Could you check a few things on this model? Use its own coordinates, in mm. A direction names the side the tool comes from. Give positions to 0.01 mm unless a question says otherwise; leave off trailing zeros. Loops run counter-clockwise (first coordinate to the right, second up) from the corner with the lowest first, then second, coordinate; pieces in that order, holes last. Notation, with made-up numbers: (-34.5, 64) - (-8.5, 64) arc R15 ccw to (-8.5, 77) - close; hole circle Ø2 at (79, 30). An arc over 180 degrees is marked (long way). One line per item, written item: value. Start each with the question number.
Q1. If I drill on line 1 (Y direction, x = -8, z = 16.75); line 2 (Y direction, x = 67, z = 16.25) (3 decimals); line 3 (Z direction, x = 69.5, y = 14) (3 decimals), over which ranges is the centre line in solid material (lowest first)? Write a range as from..to.
Q2. I want a section at A-A (x = -33). Please give me the cut outline in (y, z), then the cut area to 3 significant figures.
Q3. I'm going to push flat-ended pins straight in: P1, Ø9, axis at x = -65.88, y = -2.54, coming from the -Z side; P2, Ø11.5, axis at x = -3, y = 2, coming from the +Z side; P3, Ø3, axis at y = 7.5, z = 10, coming from the -X side. Where does each tip first touch, or does it pass through?
Q4. For faces 4 (the face through (-60.74, -20.54, 10.32)), 5 (the face through (63.182, -11, 10)), 6 (the face through (0, 0, 3.429)), 7 (the face through (-72, 16, 3.175)), 8 (the face through (70, 10.033, 10)), which set-ups out of +Z, -Z, +X, -X, +Y, -Y let a thin tool reach every point of the face, with its end or its side?
Q5. I want a section at B-B (y = -18). Please give me the cut outline in (x, z) (3 decimals), then the cut area to 3 significant figures.
Q6. If we mould it in two halves opening along X, with no side actions, what happens to faces 1 (the face through (-63.182, -12, 10)), 2 (the face through (-70, 10.033, 10)), 3 (the face through (2, 19.494, 10))? For each: released by +X, released by -X, zero draft, split by the parting line, or undercut.
Q7. I want a section at D-D (y = 17). Please give me the cut outline in (x, z) (3 decimals), then the cut area to 3 significant figures.
Q8. I want a section at C-C (z = 9.5). Count the separate pieces of the cut face and the enclosed holes in it, then the cut area to 3 significant figures.
```python
from build123d import *

# Parameters (mm, degrees)
F1_DEPTH       = 17.272
F3_DEPTH       = 13.843
F5_DEPTH       = 14.097
F7_D           = 6.858
F7_CBORE_D     = 10.033
F7_CBORE_DEPTH = 3.048


# Not quite as in the source:
# - a feature names something its author has since deleted; it is built from what else it names


with BuildPart() as f1:
    # F0 (on Top) → F1 (new body)
    with BuildSketch(Plane.XY):
        with BuildLine():
            Line((68.0447455007, 22.86), (-68.0447455007, 22.86))
            ThreePointArc((-68.0447455007, 22.86), (-75.0673121338, 19.7699967275), (-77.5335, 12.5048415503))
            Line((-77.5335, 12.5048415503), (-75.2001773438, -14.1651584497))
            ThreePointArc((-75.2001773438, -14.1651584497), (-72.146419572, -20.3575666331), (-65.7114228444, -22.86))
            Line((-65.7114228444, -22.86), (70.3780681569, -22.86))
            ThreePointArc((70.3780681569, -22.86), (77.40063479, -19.7699967275), (79.8668226562, -12.5048415503))
            Line((79.8668226562, -12.5048415503), (77.5335, 14.1651584497))
            ThreePointArc((77.5335, 14.1651584497), (74.4797422282, 20.3575666331), (68.0447455007, 22.86))
        make_face()
    extrude(amount=F1_DEPTH)

    # F2 (on face) → F3 (cut)
    with BuildSketch(Plane.XY.offset(17.272)):
        with BuildLine():
            Line((56.1975, 19.4945), (-54.61, 19.4945))
            ThreePointArc((-54.61, 19.4945), (-57.9775960454, 18.0995960454), (-59.3725, 14.732))
            Line((-59.3725, 14.732), (-59.3725, -14.732))
            ThreePointArc((-59.3725, -14.732), (-57.9775960454, -18.0995960454), (-54.61, -19.4945))
            Line((-54.61, -19.4945), (56.1975, -19.4945))
            ThreePointArc((56.1975, -19.4945), (59.5650960454, -18.0995960454), (60.96, -14.732))
            Line((60.96, -14.732), (60.96, 14.732))
            ThreePointArc((60.96, 14.732), (59.5650960454, 18.0995960454), (56.1975, 19.4945))
        make_face()
    extrude(amount=-F3_DEPTH, mode=Mode.SUBTRACT)

    # F4 (on face) → F5 (cut)
    with BuildSketch(Plane.XY.offset(17.272)):
        with BuildLine():
            Line((-76.239581844, -2.2847106486), (-77.4044675129, 11.0299934736))
            ThreePointArc((-77.4044675129, 11.0299934736), (-77.4182058621, 11.1343465964), (-77.4227969589, 11.2395))
            Line((-77.4227969589, 11.2395), (-77.5335, 12.5048415503))
            ThreePointArc((-77.5335, 12.5048415503), (-77.0333154818, 16.4863861544), (-74.9377505887, 19.9085915493))
            ThreePointArc((-74.9377505887, 19.9085915493), (-71.7938897692, 22.0911145638), (-68.0447455007, 22.86))
            Line((-68.0447455007, 22.86), (-80.5285722017, 22.86))
            Line((-80.5285722017, 22.86), (-80.5285722017, -22.86))
            Line((-80.5285722017, -22.86), (-65.7114228444, -22.86))
            ThreePointArc((-65.7114228444, -22.86), (-72.146419572, -20.3575666331), (-75.2001773438, -14.1651584497))
            Line((-75.2001773438, -14.1651584497), (-76.1550120261, -3.2513480896))
            ThreePointArc((-76.1550120261, -3.2513480896), (-76.2140031856, -2.7694909766), (-76.239581844, -2.2847106486))
        make_face()
        with BuildLine():
            Line((-77.5335, 12.5048415503), (-77.4227969589, 11.2395))
            ThreePointArc((-77.4227969589, 11.2395), (-77.0694212904, 12.0926243315), (-76.2162969589, 12.446))
            Line((-76.2162969589, 12.446), (-70.4215, 12.446))
            ThreePointArc((-70.4215, 12.446), (-67.1195, 15.748), (-70.4215, 19.05))
            Line((-70.4215, 19.05), (-74.5701236506, 19.05))
            ThreePointArc((-74.5701236506, 19.05), (-75.0371164274, 19.358045639), (-74.9377505887, 19.9085915493))
            ThreePointArc((-74.9377505887, 19.9085915493), (-77.0333154818, 16.4863861544), (-77.5335, 12.5048415503))
        make_face()
        with BuildLine():
            Line((-63.1825, 3.81), (-63.1825, 10.033))
            Line((-63.1825, 10.033), (-76.2162969589, 10.033))
            ThreePointArc((-76.2162969589, 10.033), (-76.9918202099, 10.3152673794), (-77.4044675129, 11.0299934736))
            Line((-77.4044675129, 11.0299934736), (-76.239581844, -2.2847106486))
            ThreePointArc((-76.239581844, -2.2847106486), (-75.3866698867, 1.2003753653), (-72.9243249481, 3.81))
            Line((-72.9243249481, 3.81), (-63.1825, 3.81))
        make_face()
        with BuildLine():
            ThreePointArc((-72.7051694123, -8.255), (-74.9990780637, -6.1454708758), (-76.1550120261, -3.2513480896))
            Line((-76.1550120261, -3.2513480896), (-75.2001773438, -14.1651584497))
            ThreePointArc((-75.2001773438, -14.1651584497), (-72.146419572, -20.3575666331), (-65.7114228444, -22.86))
            Line((-65.7114228444, -22.86), (-55.0545, -22.86))
            ThreePointArc((-55.0545, -22.86), (-60.8018639175, -20.4793639175), (-63.1825, -14.732))
            Line((-63.1825, -14.732), (-63.1825, -8.255))
            Line((-63.1825, -8.255), (-72.7051694123, -8.255))
        make_face()
        with BuildLine():
            ThreePointArc((63.1825, -14.732), (60.8018639175, -20.4793639175), (55.0545, -22.86))
            Line((55.0545, -22.86), (70.3780681569, -22.86))
            ThreePointArc((70.3780681569, -22.86), (77.40063479, -19.7699967275), (79.8668226562, -12.5048415503))
            Line((79.8668226562, -12.5048415503), (78.9578200825, -2.114894589))
            ThreePointArc((78.9578200825, -2.114894589), (77.1524285249, -6.5300931701), (72.7051694123, -8.255))
            Line((72.7051694123, -8.255), (63.1825, -8.255))
            Line((63.1825, -8.255), (63.1825, -14.732))
        make_face()
        with BuildLine():
            ThreePointArc((77.5335, 14.1651584497), (76.7244498583, 17.2577996716), (74.9377505887, 19.9085915493))
            ThreePointArc((74.9377505887, 19.9085915493), (75.0371164274, 19.358045639), (74.5701236506, 19.05))
            Line((74.5701236506, 19.05), (70.4215, 19.05))
            ThreePointArc((70.4215, 19.05), (67.1195, 15.748), (70.4215, 12.446))
            Line((70.4215, 12.446), (76.2162969589, 12.446))
            ThreePointArc((76.2162969589, 12.446), (77.4227969589, 11.2395), (76.2162969589, 10.033))
            Line((76.2162969589, 10.033), (63.1825, 10.033))
            Line((63.1825, 10.033), (63.1825, 3.81))
            Line((63.1825, 3.81), (72.9243249481, 3.81))
            ThreePointArc((72.9243249481, 3.81), (76.8450400591, 2.3627819378), (78.8851888528, -1.2847158349))
            Line((78.8851888528, -1.2847158349), (77.5335, 14.1651584497))
        make_face()
    extrude(amount=-F5_DEPTH, mode=Mode.SUBTRACT)

    # F7 (through all)
    with Locations(Plane(origin=(0, 0, 0), x_dir=(1, 0, 0), z_dir=(0, 0, -1))):
        with Locations((72.23125, 2.54), (-65.88125, 2.54)):
            CounterBoreHole(F7_D / 2, F7_CBORE_D / 2, F7_CBORE_DEPTH)


solid = f1.part
```
Worked answers:
1. line 1: y = -22.86..-19.49, 19.49..22.86
1. line 2: y = -8.255..3.81, 10.033..22.86
1. line 3: z = 0..3.175
2. outline: (-22.86, 0) - (22.86, 0) - (22.86, 17.27) - (19.49, 17.27) - (19.49, 3.43) - (-19.49, 3.43) - (-19.49, 17.27) - (-22.86, 17.27) - close
2. area: 250 mm²
3. P1: stops at z = 3.05
3. P2: stops at z = 3.43
3. P3: stops at x = -63.18
4. face 4: +Z, -X, -Y
4. face 5: +Z, +X, -Y
4. face 6: +Z
4. face 7: +Z, -X
4. face 8: +Z, +X
5. outline: (-74.016, 0) - (78.682, 0) - (78.682, 3.175) - (62.497, 3.175) - (62.497, 17.272) - (59.662, 17.272) - (59.662, 3.429) - (-58.074, 3.429) - (-58.074, 17.272) - (-62.497, 17.272) - (-62.497, 3.175) - (-74.016, 3.175) - close
5. area: 617 mm²
6. face 1: released by -X
6. face 2: zero draft
6. face 3: undercut
7. outline: (-76.836, 0) - (76.836, 0) - (76.836, 3.175) - (67.366, 3.175) - (67.366, 17.272) - (60.385, 17.272) - (60.385, 3.429) - (-58.798, 3.429) - (-58.798, 17.272) - (-67.366, 17.272) - (-67.366, 3.175) - (-76.836, 3.175) - close
7. area: 737 mm²
8. separate pieces: 1
8. enclosed holes: 3
8. area: 1,530 mm²
